Autodesk Inventor part; units mm, degrees
ref_plane "YZ Plane" through (0, 0, 0) normal (1, 0, 0) x (0, 1, 0)
ref_plane "XZ Plane" through (0, 0, 0) normal (0, 1, 0) x (-1, 0, 0)
ref_plane "XY Plane" through (0, 0, 0) normal (0, 0, 1) x (1, 0, 0)
sketch "スケッチ1" plane through (0, 0, 0) normal (0, 1, 0) x (-1, 0, 0)
  line L0 (0, 0) -> (-64.0652, 0) construction
  circle A0 centre (-28.65, 0) radius 2.85
  line L1 (-23.65, -3.5) -> (-28.65, -3.5)
  line L2 (-28.65, -3.5) -> (-28.65, 3.5)
  line L3 (-28.65, 3.5) -> (-23.65, 3.5)
  line L4 (-23.65, 3.5) -> (-23.65, -3.5)
  line L5 (0, -4.9) -> (0, 4.9)
  point P0 (-28.65, 2.85)
  point P1 (-28.65, -2.85)
  dimension "P_DIA" = 5.7
  dimension "P_D1" = 28.65
  dimension "d2" = 7
  dimension "d3" = 5
revolve "リム" add sketch "スケッチ1" angle 360 about axis through (0, 0, -10) along (0, 0, 1) contours A0 L2 L3 L4 L1
sketch "スケッチ3" plane through (0, 0, 3.5) normal (0, 0, 1) x (1, 0, 0)
  line L0 (-5, 2.8868) -> (0, 5.7735)
  line L1 (0, 5.7735) -> (5, 2.8868)
  line L2 (5, 2.8868) -> (5, -2.8868)
  line L3 (5, -2.8868) -> (0, -5.7735)
  line L4 (0, -5.7735) -> (-5, -2.8868)
  line L5 (-5, -2.8868) -> (-5, 2.8868)
  point P0 (0, 0)
  point P1 (0, 0)
  dimension "HUB_DIA" = 10
extrude "ハブ" add sketch "スケッチ3" against normal up to surface (7 mm away)
sketch "スケッチ4" plane through (0, 0, 3.5) normal (0, 0, 1) x (1, 0, 0)
  line L0 (-0.8, 0) -> (0.8, 0)
  line L1 (0.8, 0) -> (0.8, 23.65)
  line L2 (0.8, 23.65) -> (-0.8, 23.65)
  line L3 (-0.8, 23.65) -> (-0.8, 0)
  circle A0 centre (0, 0) radius 23.65
  point P0 (0, 23.65)
  dimension "SPOKE_THIN" = 1.6
extrude "スポーク" add sketch "スケッチ4" against normal up to surface (7 mm away) contours L3 A0 L1 L0 | L3 L2 A0 | A0 L2 L1 picked at (0, 7.8833)
pattern_circular "円形状パターン1" count 6 over 360 about axis through (0, 0, -10) along (0, 0, 1) of "スポーク"
sketch "スケッチ5" plane through (0, 0, 3.5) normal (0, 0, 1) x (1, 0, 0)
  line L0 (-2.5, 1.575) -> (2.5, 1.575)
  line L1 (2.5, 1.575) -> (2.5, -1.575)
  line L2 (2.5, -1.575) -> (-2.5, -1.575)
  line L3 (-2.5, -1.575) -> (-2.5, 1.575)
  point P0 (0, 0)
  point P1 (0, 1.575)
  point P2 (-2.5, 0)
  dimension "d15" = 5
  dimension "d16" = 3.15
extrude "軸穴" cut sketch "スケッチ5" against normal through all
properties part number "Wheel-D63C"
Could you check a few things on this model? Use its own coordinates, in mm. Give positions to 0.01 mm unless a question says otherwise; leave off trailing zeros. Write each loop counter-clockwise with the first axis right and the second up, starting at its lowest first coordinate (ties: lowest second). Pieces come first, ordered by that corner, then holes. Notation, with made-up numbers: (56.25, 55.25) - (107.25, 55.25) arc R20 cw to (107.25, 92.25) - close; hole circle Ø10 at (39.25, -28.75). An arc over 180 degrees is marked (long way). Use CSV: the item, a comma, the result in double quotes. Start each with the question number.
Item 1: I want a section at B-B, the plane x = 0. Please give me the cut outline in (y, z) (3 decimals).
Item 2: If we mould it in two halves opening along X, with no side actions, what happens to faces 1 (the face through (0, 2, -3.5)), 2 (the face through (0, -1.575, 0)), 3 (the face through (27.327, 8.606, 3.18))? For each: pulls with the +X half, pulls with the -X half, needs draft (parallel to the pull), parting line crosses it, or undercut.
Item 3: I want a section at A-A, the plane y = 0. Please give me the cut outline in (x, z).
Item 4: I'm going to push flat-ended pins straight in: pin 1 (1.5 mm diameter, centred on y = 14, z = -1.5, fed in from -X); pin 2 (2.5 mm diameter, centred on y = -0.5, z = 0.5, fed in from -X); pin 3 (2 mm diameter, centred on y = 10.5, z = 1.5, fed in from +X); pin 4 (5 mm diameter, centred on x = -4.5, y = -17.5, fed in from -Z). Where does each tip first touch, or does it pass through?
Item 5: If I drill on line 1 along X through (y, z) = (2, -1); line 2 along X through (y, z) = (10, -1.75); line 3 along X through (y, z) = (-11, -1.5), over which ranges is the centre line in solid material (lowest first)?
Item 6: I want a section at C-C, the plane z = -1.75. Give the number of separate pieces and of enclosed holes in the cut face, then the cut area to 3 significant figures.
Findings:
1,outline,"(-28.65, -3.5) - (-1.575, -3.5) - (-1.575, 3.5) - (-28.65, 3.5) - (-28.65, 2.85) arc R2.85 cw to (-28.65, -2.85) - close; (1.575, -3.5) - (28.65, -3.5) - (28.65, -2.85) arc R2.85 cw to (28.65, 2.85) - (28.65, 3.5) - (1.575, 3.5) - close"
2,face 1,"needs draft"
2,face 2,"undercut"
2,face 3,"parting line crosses it"
3,outline,"(-28.65, -3.5) - (-23.65, -3.5) - (-23.65, 3.5) - (-28.65, 3.5) - (-28.65, 2.85) arc R2.85 cw to (-28.65, -2.85) - close; (-5, -3.5) - (-2.5, -3.5) - (-2.5, 3.5) - (-5, 3.5) - close; (2.5, -3.5) - (5, -3.5) - (5, 3.5) - (2.5, 3.5) - close; (23.65, -3.5) - (28.65, -3.5) - (28.65, -2.85) arc R2.85 cw to (28.65, 2.85) - (28.65, 3.5) - (23.65, 3.5) - close"
4,pin 1,"stops at x = -23.06"
4,pin 2,"stops at x = -26.4"
4,pin 3,"stops at x = 25.22"
4,pin 4,"passes through"
5,line 1,"x = -25.9 to -23.57, -5.06 to 5.06, 23.57 to 25.9"
5,line 2,"x = -24.43 to -21.43, -18.92 to -15.72, -0.8 to 0.8, 15.72 to 18.92, 21.43 to 24.43"
5,line 3,"x = -23.81 to -20.94, -20.65 to -17.45, -0.8 to 0.8, 17.45 to 20.65, 20.94 to 23.81"
6,separate pieces,"1"
6,enclosed holes,"7"
6,area,"677 mm2"
